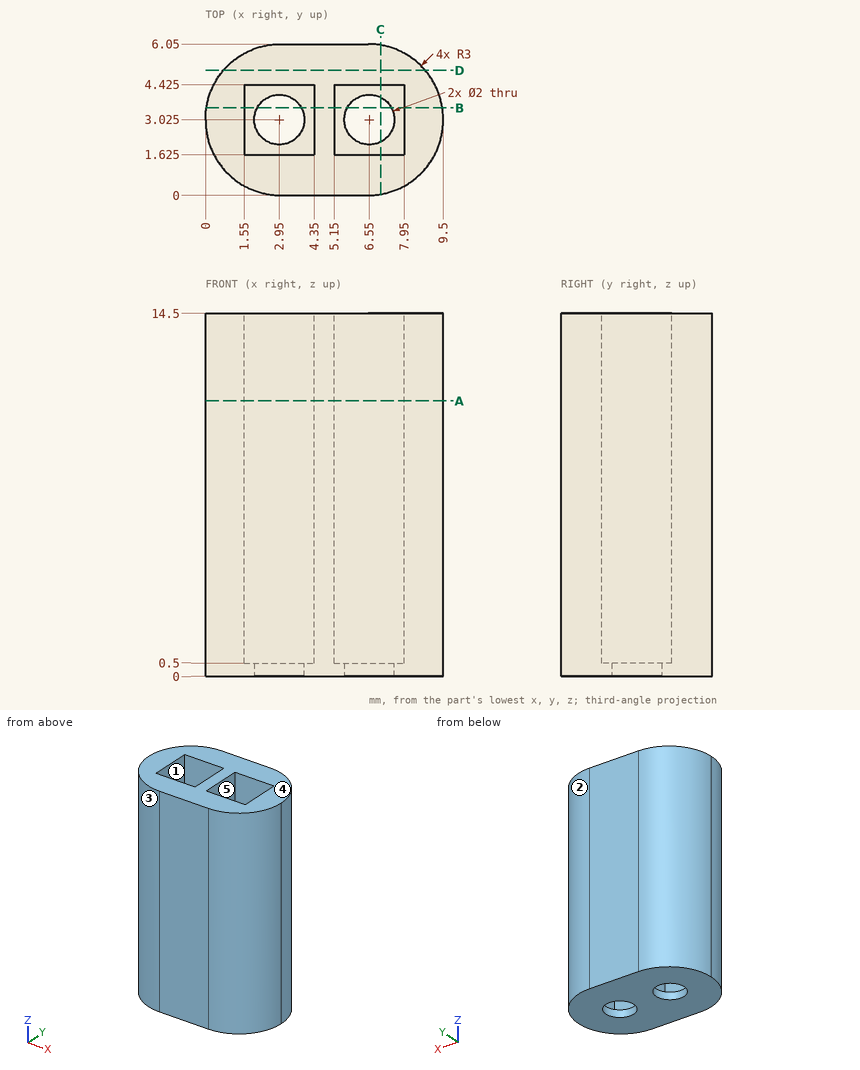
Geometry check sheet. Reference: drawing and pictorial views, mm from the part's lowest x, y, z. A direction names the side the tool comes from. Coordinates: 2 decimals unless noted, no trailing zeros. Order: outer loops, then holes, each group sorted by start corner. A loop starts at its lowest first (then second) coordinate and runs counter-clockwise, first axis right, second up.
Item 1: Section check A-A, the plane z = 11. Enter the section's corners in (x, y) (3 decimals), then the cut area to 3 significant figures.
Filled in:
outline: (0, 3) arc R3 ccw to (3, 0) - (6.5, 0) arc R3 ccw to (9.5, 3) - (9.5, 3.05) arc R3 ccw to (6.5, 6.05) - (3, 6.05) arc R3 ccw to (0, 3.05) - close; hole (1.55, 1.625) - (4.35, 1.625) - (4.35, 4.425) - (1.55, 4.425) - close; hole (5.15, 1.625) - (7.95, 1.625) - (7.95, 4.425) - (5.15, 4.425) - close
area: 34.1 mm2
Item 2: Material ranges on L1, parallel to Y at x = 2.95, z = 0.2 (3 decimals); L2, parallel to Y at x = 5.25, z = 14.25 (3 decimals); L3, parallel to X at y = 1.75, z = 3.5, recorded low to high.
Filled in:
L1: y = 0 to 2.025, 4.025 to 6.05
L2: y = 0 to 1.625, 4.425 to 6.05
L3: x = 0.27 to 1.55, 4.35 to 5.15, 7.95 to 9.23
Item 3: Section check B-B, the plane y = 3.5. Enter the section's corners in (x, z), then the cut area to 3 significant figures.
Filled in:
outline: (0.03, 0) - (2.07, 0) - (2.07, 0.5) - (1.55, 0.5) - (1.55, 14.5) - (0.03, 14.5) - close; (3.83, 0) - (5.67, 0) - (5.67, 0.5) - (5.15, 0.5) - (5.15, 14.5) - (4.35, 14.5) - (4.35, 0.5) - (3.83, 0.5) - close; (7.43, 0) - (9.47, 0) - (9.47, 14.5) - (7.95, 14.5) - (7.95, 0.5) - (7.43, 0.5) - close
area: 56.6 mm2
Item 4: Access from +Z, -Z, +X, -X, +Y, -Y to the whole of each face (thin tool, end or side, straight path). Record for the marked faces 1 and 2.
Filled in:
face 1: +Z
face 2: +Z, -Z, +X, +Y
Item 5: Section check C-C, the plane x = 7. Enter the section's corners in (y, z) (3 decimals).
Filled in:
outline: (0.042, 0) - (2.132, 0) - (2.132, 0.5) - (1.625, 0.5) - (1.625, 14.5) - (0.042, 14.5) - close; (3.918, 0) - (6.008, 0) - (6.008, 14.5) - (4.425, 14.5) - (4.425, 0.5) - (3.918, 0.5) - close
Item 6: Depth check by flat-ended pin: pin 1 (3 mm diameter, centred on y = 5, z = 6, fed in from +X). Enter the tip coordinate at first touch or a pass-through.
Filled in:
pin 1: stops at x = 9.47
Item 7: Release check for a two-part mould opening along X. For the marked faces 3, 4 and 5 record: +X half, -X half, draft (parallel to the pull), parting line (faces both ways), or undercut.
Filled in:
face 3: -X half
face 4: draft
face 5: undercut
Item 8: Section check D-D, the plane y = 5. Enter the section's corners in (x, z), then the cut area to 3 significant figures.
Filled in:
outline: (0.72, 0) - (8.78, 0) - (8.78, 14.5) - (0.72, 14.5) - close
area: 117 mm2
